Geometry check sheet. Reference: the model listing, model coordinates, mm. Face numbers are marked on the shaded views. A direction names the side the tool comes from. Coordinates: 2 decimals unless noted, no trailing zeros. Loops run counter-clockwise (first coordinate to the right, second up) from the corner with the lowest first, then second, coordinate; pieces in that order, holes last. Notation, with made-up numbers: (30.25, 58.25) - (40.25, 58.25) arc R18 ccw to (40.25, 66.25) - close; hole circle Ø5 at (66.5, 16). An arc over 180 degrees is marked (long way). Write item = value, one per line. Start each with the question number.
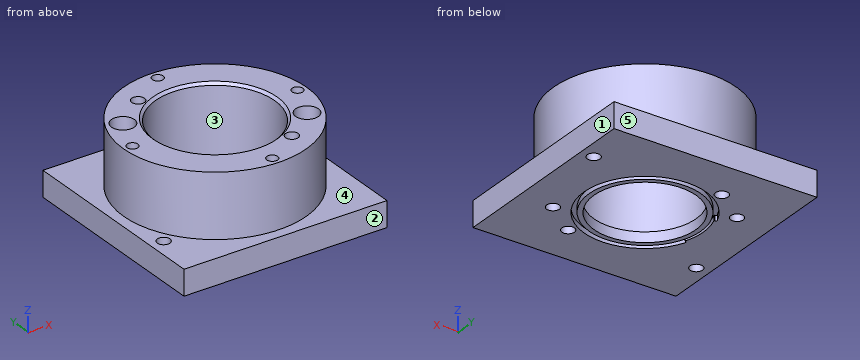
from build123d import *

# Parameters (mm, degrees)
SKIZZE1_W                                            = 80
SKIZZE1_H                                            = 80
AUFSATZ_LINEAR_AUSTRAGEN1_DEPTH                      = 10
SKIZZE16_R                                           = 20.1
SCHNITT_LINEAR_AUSTRAGEN1_DEPTH                      = 11
SKIZZE17_R                                           = 36
SKIZZE17_R_2                                         = 23.5
AUFSATZ_LINEAR_AUSTRAGEN2_DEPTH                      = 25
KREISMUSTER1_COUNT                                   = 4
FASE1_SIZE                                           = 1
F_5_0_5_DURCHMESSER_BOHRUNG1_D                       = 5
STIRNSENKUNG_F_R_M5_ZYLINDERSCHRAUBE_MIT_D           = 5
STIRNSENKUNG_F_R_M5_ZYLINDERSCHRAUBE_MIT_CBORE_D     = 9
STIRNSENKUNG_F_R_M5_ZYLINDERSCHRAUBE_MIT_CBORE_DEPTH = 7
SKIZZE39_R                                           = 23.5
SKIZZE39_R_2                                         = 20.1
SCHNITT_LINEAR_AUSTRAGEN2_DEPTH                      = 6
SKIZZE40_R                                           = 24
SKIZZE40_R_2                                         = 22
SCHNITT_LINEAR_AUSTRAGEN3_DEPTH                      = 2
AUFSATZ_LINEAR_AUSTRAGEN3_DEPTH                      = 2
SCHNITT_LINEAR_AUSTRAGEN4_DEPTH                      = 2


with BuildPart() as part:
    # Skizze1 → Aufsatz-Linear austragen1 (new body)
    with BuildSketch(Plane.XY):
        Rectangle(SKIZZE1_W, SKIZZE1_H)
    extrude(amount=AUFSATZ_LINEAR_AUSTRAGEN1_DEPTH)

    # Skizze16 → Schnitt-Linear austragen1 (cut, through all)
    with BuildSketch(Plane.XY.offset(10)):
        Circle(SKIZZE16_R)
    extrude(amount=-SCHNITT_LINEAR_AUSTRAGEN1_DEPTH, mode=Mode.SUBTRACT)

    # Skizze17 → Aufsatz-Linear austragen2 (add)
    with BuildSketch(Plane.XY.offset(10)):
        Circle(SKIZZE17_R)
        Circle(SKIZZE17_R_2, mode=Mode.SUBTRACT)
    extrude(amount=AUFSATZ_LINEAR_AUSTRAGEN2_DEPTH)

    # Skizze21 → Ø4.3 (4.3) Durchmesser Bohrung1 (revolve, cut)
    with BuildSketch(Plane(origin=(0, 32.5, 35), x_dir=(0, -1, 0), z_dir=(1, 0, 0))):
        Polygon((0, 0), (0, 16.291850331), (2.15, 15), (2.15, 0), align=None)
    f_4_3_4_3_durchmesser_bohrung1 = revolve(axis=Axis((0, 32.5, 41.35), (0, 0, -1)), mode=Mode.SUBTRACT)

    # Kreismuster1: Ø4.3 (4.3) Durchmesser Bohrung1 ×4 about axis
    kreismuster1_axis = Axis((0, 0, 0), (0, 0, 1))
    for i in range(1, KREISMUSTER1_COUNT):
        add(f_4_3_4_3_durchmesser_bohrung1.rotate(kreismuster1_axis, i * 360 / KREISMUSTER1_COUNT), mode=Mode.SUBTRACT)

    # Fase1
    fase1_edges = [part.edges().sort_by_distance(p)[0] for p in [
        (-23.5, 0, 35),
    ]]
    chamfer(fase1_edges, length=FASE1_SIZE)

    # Ø5.0 (5) Durchmesser Bohrung1 (through all)
    with Locations(Plane(origin=(0, 0, 0), x_dir=(-1, 0, 0), z_dir=(0, 0, -1))):
        with Locations((34.715275678, -20.859042034), (-13.75, -23.815698604), (13.75, 23.815698604), (-34.715275678, 20.859042034)):
            Hole(F_5_0_5_DURCHMESSER_BOHRUNG1_D / 2)

    # Stirnsenkung für M5 Zylinderschraube mit Innensechskant1 (through all)
    with Locations(Plane.XY.offset(35)):
        with Locations((-26.488427786, 14.084146884), (26.488427786, -14.084146884)):
            CounterBoreHole(STIRNSENKUNG_F_R_M5_ZYLINDERSCHRAUBE_MIT_D / 2, STIRNSENKUNG_F_R_M5_ZYLINDERSCHRAUBE_MIT_CBORE_D / 2, STIRNSENKUNG_F_R_M5_ZYLINDERSCHRAUBE_MIT_CBORE_DEPTH)

    # Skizze39 → Schnitt-Linear austragen2 (cut)
    with BuildSketch(Plane.XY.offset(10)):
        Circle(SKIZZE39_R)
        Circle(SKIZZE39_R_2, mode=Mode.SUBTRACT)
    extrude(amount=-SCHNITT_LINEAR_AUSTRAGEN2_DEPTH, mode=Mode.SUBTRACT)

    # Skizze40 → Schnitt-Linear austragen3 (cut)
    with BuildSketch(Plane(origin=(0, 0, 0), x_dir=(-1, 0, 0), z_dir=(0, 0, -1))):
        Circle(SKIZZE40_R)
        Circle(SKIZZE40_R_2, mode=Mode.SUBTRACT)
    extrude(amount=-SCHNITT_LINEAR_AUSTRAGEN3_DEPTH, mode=Mode.SUBTRACT)

    # Skizze41 → Aufsatz-Linear austragen3 (add)
    with BuildSketch(Plane(origin=(0, 0, 2), x_dir=(-1, 0, 0), z_dir=(0, 0, -1))):
        with BuildLine():
            Line((21.16903947, -8.992508512), (22.25162445, -8.992508512))
            ThreePointArc((22.25162445, -8.992508512), (24.003029137, 0.007491459), (22.251624746, 9.007491488))
            Line((22.251624746, 9.007491488), (21.169039781, 9.007491488))
            ThreePointArc((21.169039781, 9.007491488), (23.003029137, 0.007491456), (21.16903947, -8.992508512))
        make_face()
    extrude(amount=AUFSATZ_LINEAR_AUSTRAGEN3_DEPTH)

    # Skizze42 → Schnitt-Linear austragen4 (cut)
    with BuildSketch(Plane(origin=(0, 0, 0), x_dir=(-1, 0, 0), z_dir=(0, 0, -1))):
        with BuildLine():
            Line((21.431430131, -8.305164585), (21.16903947, -8.992508512))
            Line((21.16903947, -8.992508512), (21.324473431, -8.992508512))
            ThreePointArc((21.324473431, -8.992508512), (22.202579979, -9.084742871), (21.788048941, -8.305164585))
            Line((21.788048941, -8.305164585), (21.431430131, -8.305164585))
        make_face()
        with BuildLine():
            Line((21.782114297, 8.319835415), (21.431430131, 8.319835415))
            Line((21.431430131, 8.319835415), (21.169039781, 9.007491488))
            Line((21.169039781, 9.007491488), (21.318665057, 9.007491488))
            ThreePointArc((21.318665057, 9.007491488), (22.196739451, 9.099274106), (21.782114297, 8.319835415))
        make_face()
    extrude(amount=-SCHNITT_LINEAR_AUSTRAGEN4_DEPTH, mode=Mode.SUBTRACT)


solid = part.part
(1) Scan lines: line 1 (X direction, y = 15, z = 26); line 2 (X direction, y = 17, z = 29); line 3 (X direction, y = -1.5, z = 33). Record each from-to range of solid material in increasing order.
(2) Draft check along Y on the marked faces 1, 2 and 3. Enter one of: pulls with the +Y half, pulls with the -Y half, needs draft (parallel to the pull), parting line crosses it, or undercut.
(3) Sectioned sample at B-B on z = 8. Enter the section's corners in (x, y), plus the area to 3 significant figures.
(4) Tool access check on the marked faces 4 and 5. Record the directions out of +Z, -Z, +X, -X, +Y, -Y that give a thin tool (end or side, any length) a straight path to the whole face; none if there is none.
(5) Sectioned sample at A-A on z = 21. Count the separate pieces of the cut face and the enclosed holes in it, plus the area to 3 significant figures.
(6) Depth check by flat-ended pin: pin 1 (4 mm diameter, centred on x = -0.5, y = -26.5, fed in from -Z); pin 2 (6 mm diameter, centred on x = 26.49, y = -14.08, fed in from +Z); pin 3 (3 mm diameter, centred on x = 34.72, y = 20.86, fed in from +Z); pin 4 (3.5 mm diameter, centred on x = -32.5, y = 0, fed in from +Z). Enter the tip coordinate at first touch or a pass-through.
Working result:
q1.line_1 = -32.73 to -28.81, -24.16 to -18.09, 18.09 to 32.73
q1.line_2 = -31.73 to -29.92, -23.06 to -16.22, 16.22 to 31.73
q1.line_3 = -35.97 to -34.04, -30.96 to -23.45, 23.45 to 30.96, 34.04 to 35.97
q2.face_1 = needs draft
q2.face_2 = pulls with the -Y half
q2.face_3 = undercut
q3.outline = (-40, -40) - (40, -40) - (40, 40) - (-40, 40) - close; hole circle Ø5 at (-34.72, -20.86); hole circle Ø5 at (-26.49, 14.08); hole circle Ø47 at (0, 0); hole circle Ø5 at (-13.75, 23.82); hole circle Ø5 at (13.75, -23.82); hole circle Ø5 at (26.49, -14.08); hole circle Ø5 at (34.72, 20.86)
q3.area = 4,550 mm2
q4.face_4 = +Z
q4.face_5 = +Z, -Z, +X, -X, +Y
q5.separate_pieces = 1
q5.enclosed_holes = 9
q5.area = 2,200 mm2
q6.pin_1 = 0
q6.pin_2 = 28
q6.pin_3 = through
q6.pin_4 = 19.76
